from build123d import *

# Parameters (mm, degrees)
BOSS_EXTRUDE2_DEPTH = 33.5
SKETCH2_R           = 10
CUT_EXTRUDE1_DEPTH  = 49.787805854


with BuildPart() as part:
    # Sketch1 → Boss-Extrude2 (new body)
    with BuildSketch(Plane(origin=(0, 0, 0), x_dir=(1, 0, 0), z_dir=(0, 1, 0))):
        with BuildLine():
            Line((0, 0), (0, 13))
            Line((0, 13), (20, 13))
            ThreePointArc((20, 13), (33, 0), (20, -13))
            Line((20, -13), (0, -13))
            Line((0, -13), (0, 0))
        make_face()
    extrude(amount=-BOSS_EXTRUDE2_DEPTH)

    # Sketch2 → Cut-Extrude1 (cut, through all)
    with BuildSketch(Plane(origin=(0, 0, 0), x_dir=(1, 0, 0), z_dir=(0, 1, 0))):
        with Locations(Location((20, 0, 0), (0, 0, 270))):
            Circle(SKETCH2_R)
    extrude(amount=-CUT_EXTRUDE1_DEPTH, mode=Mode.SUBTRACT)


solid = part.part
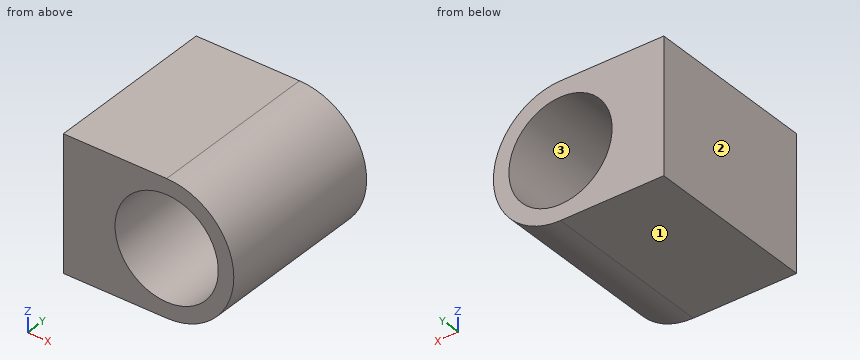
For this review, take the finished solid that the model builds, in its own axes (mm). Face numbers are marked on the shaded views. Coordinates: 2 decimals unless noted, no trailing zeros. Order: outer loops, then holes, each group sorted by start corner. A loop starts at its lowest first (then second) coordinate and runs counter-clockwise, first axis right, second up. Notation, with made-up numbers: (6.25, 35.25) - (28.25, 35.25) arc R27 cw to (28.25, 61.25) - close; hole circle Ø2 at (-12.5, -3.5). An arc over 180 degrees is marked (long way). Answer as CSV lines item,"result". Start each with the question number.
1) Add section A-A (z = 0). State the section outline as (x, y) points, then the cut area to 4 significant figures.
2) Insertion check: P1, Ø5, axis at x = 23.5, y = -5.5, coming from the -Z side; P2, Ø8, axis at y = -29, z = 10, coming from the +X side. Each pin has a flat end and moves straight along its axis. Give the tip position at first contact, or say it passes through.
3) To check wall thickness, follow line 1 along X through (y, z) = (-8.5, 0); line 2 along X through (y, z) = (-1.5, 4.25); line 3 along Z through (x, y) = (12, -32). State the ranges of each line that lie inside material, in increasing order. Write a range as [from, to].
4) Add section B-B (x = 22.5). State the section outline as (y, z) points, then the cut area to 3 significant figures.
5) Add section C-C (y = -29.5). State the section outline as (x, z) points.
6) Draft analysis for pull direction Z (two halves, no side actions). For the marked faces 1, 2 and 3, state which applies: +Z half, -Z half, draft (parallel to the pull), parting line (faces both ways), or undercut.
Result:
1,outline,"(0, -33.5) - (10, -33.5) - (10, 0) - (0, 0) - close; (30, -33.5) - (33, -33.5) - (33, 0) - (30, 0) - close"
1,area,"435.5 mm^2"
2,P1,"z = -12.96"
2,P2,"x = 31.53"
3,line 1,"[0, 10], [30, 33]"
3,line 2,"[0, 10.95], [29.05, 32.29]"
3,line 3,"[-13, -6], [6, 13]"
4,outline,"(-33.5, -12.76) - (0, -12.76) - (0, -9.68) - (-33.5, -9.68) - close; (-33.5, 9.68) - (0, 9.68) - (0, 12.76) - (-33.5, 12.76) - close"
4,area,"206 mm^2"
5,outline,"(0, -13) - (20, -13) arc R13 ccw to (20, 13) - (0, 13) - close; hole circle Ø20 at (20, 0)"
6,face 1,"-Z half"
6,face 2,"draft"
6,face 3,"undercut"
